from build123d import *

# Parameters (mm, degrees)
SKETCH1_W           = 335
SKETCH1_H           = 100
SKETCH1_W_2         = 325
SKETCH1_H_2         = 92.5
BOSS_EXTRUDE1_DEPTH = 10
FILLET1_R           = 10
BOSS_EXTRUDE2_DEPTH = 3


with BuildPart() as part:
    # Sketch1 → Boss-Extrude1 (new body)
    with BuildSketch(Plane.XY):
        Rectangle(SKETCH1_W, SKETCH1_H)
        Rectangle(SKETCH1_W_2, SKETCH1_H_2, mode=Mode.SUBTRACT)
    extrude(amount=-BOSS_EXTRUDE1_DEPTH)

    # Fillet1
    fillet1_edges = [part.edges().sort_by_distance(p)[0] for p in [
        (167.5, -50, -5),
        (-167.5, -50, -5),
        (-167.5, 50, -5),
        (167.5, 50, -5),
    ]]
    fillet(fillet1_edges, radius=FILLET1_R)

    # Sketch2 → Boss-Extrude2 (add)
    with BuildSketch(Plane(origin=(0, 0, -10), x_dir=(-1, 0, 0), z_dir=(0, 0, -1))):
        Polygon((-162.5, -46.25), (-162.5, -36.25), (-152.5, -46.25), align=None)
        Polygon((-162.5, 46.25), (-152.5, 46.25), (-162.5, 36.25), align=None)
        Polygon((162.5, 46.25), (152.5, 46.25), (162.5, 36.25), align=None)
        Polygon((162.5, -46.25), (162.5, -36.25), (152.5, -46.25), align=None)
    extrude(amount=-BOSS_EXTRUDE2_DEPTH)


solid = part.part
Read the model definition and answer for the solid it produces. Units are mm, in the model's axes. A direction names the side the tool comes from. Give positions to 0.01 mm unless a question says otherwise; leave off trailing zeros. Loops run counter-clockwise (first coordinate to the right, second up) from the corner with the lowest first, then second, coordinate; pieces in that order, holes last. Notation, with made-up numbers: (-38, -35) -> (-33, -35) arc R23 cw to (-33, -10) -> close; hole circle Ø1 at (-40, 33.5). An arc over 180 degrees is marked (long way). Answer as CSV lines item,"result".
Item 1: Find section A-A on y = 10. Give the vertices of the cut face in (x, z), plus the area to 3 significant figures.
Returned:
outline,"(-167.5, -10) -> (-162.5, -10) -> (-162.5, 0) -> (-167.5, 0) -> close; (162.5, -10) -> (167.5, -10) -> (167.5, 0) -> (162.5, 0) -> close"
area,"100 mm²"
Item 2: Consider line 1 (Y direction, x = -53, z = -4.25); line 2 (X direction, y = 29, z = -9); line 3 (X direction, y = -41, z = -2). Determine where each line is inside the solid, lowest interval first. Write a range as [from, to].
Returned:
line 1,"y = [-50, -46.25], [46.25, 50]"
line 2,"x = [-167.5, -162.5], [162.5, 167.5]"
line 3,"x = [-167.45, -162.5], [162.5, 167.45]"
Item 3: This flat-tipped pin is pushed along its axis until it touches: pin 1 (8 mm diameter, centred on x = 157.5, y = -40, fed in from +Z). Where does it stop, or does it pass through?
Returned:
pin 1,"stops at z = -7"
Item 4: Find section B-B on x = 34. Give the vertices of the cut face in (y, z).
Returned:
outline,"(-50, -10) -> (-46.25, -10) -> (-46.25, 0) -> (-50, 0) -> close; (46.25, -10) -> (50, -10) -> (50, 0) -> (46.25, 0) -> close"
Item 5: For faces 1 (the face through (160, -43, -7)), 2 (the face through (-157.57, -41.18, -8.52)), 3 (the face through (164.49, -47.15, -5.07)), determine the directions among +Z, -Z, +X, -X, +Y, -Y from which every point of the face is accessible in a straight line to the end or side of a thin tool.
Returned:
face 1,"+Z"
face 2,"+Z, -Z"
face 3,"+Z, -Z, +X, -Y"
Item 6: Find section C-C on y = -43. Give the vertices of the cut face in (x, z).
Returned:
outline,"(-167.04, -10) -> (-155.75, -10) -> (-155.75, -7) -> (-162.5, -7) -> (-162.5, 0) -> (-167.04, 0) -> close; (155.75, -10) -> (167.04, -10) -> (167.04, 0) -> (162.5, 0) -> (162.5, -7) -> (155.75, -7) -> close"
Item 7: Determine the mould class of faces 4 (the face through (-167.5, -1, -5)), 5 (the face through (-157.43, 41.32, -8.52)), 6 (the face through (-2, -50, -5)) for opening direction Y: +Y half, -Y half, draft (parallel to the pull), parting line (faces both ways), or undercut.
Returned:
face 4,"draft"
face 5,"undercut"
face 6,"-Y half"
